Read the model definition and answer for the solid it produces. Units are mm, in the model's axes. A direction names the side the tool comes from. Coordinates: 2 decimals unless noted, no trailing zeros. Loops run counter-clockwise (first coordinate to the right, second up) from the corner with the lowest first, then second, coordinate; pieces in that order, holes last. Notation, with made-up numbers: (61, 54) -> (92, 54) arc R13 ccw to (92, 70) -> close; hole circle Ø4 at (52.25, 33.25). An arc over 180 degrees is marked (long way). Answer in a Markdown table with one row per item.
```python
from build123d import *

# Parameters (mm, degrees)
F1_DEPTH     = 20
F3_D         = 5
F5_T3_DEPTH  = 150
F5_T6_DEPTH  = 40
F5_T9_DEPTH  = 30
F5_T12_DEPTH = 25
F5_T15_DEPTH = 100
F5_T18_DEPTH = 25
F5_T21_DEPTH = 30
F5_T24_DEPTH = 40
F5_T33_DEPTH = 150
F5_T36_DEPTH = 40
F5_T39_DEPTH = 30
F5_T42_DEPTH = 25
F5_T45_DEPTH = 100
F5_T48_DEPTH = 25
F5_T51_DEPTH = 30
F5_T54_DEPTH = 40
F5_T64_DEPTH = 105
F5_T68_DEPTH = 30
F5_T74_DEPTH = 30
F5_T78_DEPTH = 105
F5_T84_DEPTH = 30
F5_T88_DEPTH = 105
F5_T94_DEPTH = 105
F5_T98_DEPTH = 30


# Not quite as in the source:
# - a fillet or chamfer that OpenCascade refuses, or shapes differently, is made with other operations: its cross-section is extruded or revolved along the edge and cut away or added


with BuildPart() as f1:
    # F0 (on Top) → F1 (new body)
    with BuildSketch(Plane.XY):
        Polygon((45.4953936456, 30), (-24.5046063544, 30), (-24.5046063544, 20), (25.4953936456, 20), (25.4953936456, 0), (45.4953936456, 0), align=None)
    extrude(amount=F1_DEPTH)

    # F3 (through all)
    with Locations(Plane.XY.offset(20)):
        with Locations((40.4953936456, 5)):
            Hole(F3_D / 2)

    # F4: F1 across face


with BuildPart() as f1_1:
    add(f1.part)
    add(f1.part.mirror(Plane(origin=(-24.5046063544, 25, 10), x_dir=(0, -1, 0), z_dir=(-1, 0, 0))))

    # F5: fillet of radius 2 on 20 edges, made by hand


with BuildPart() as f5_tool1:
    # F5_s2 → F5_t3 (new body)
    with BuildSketch(Plane.YZ.offset(-99.5046063544)):
        with BuildLine():
            ThreePointArc((30, 18), (29.4142135624, 19.4142135624), (28, 20))
            Line((28, 20), (30, 20))
            Line((30, 20), (30, 18))
        make_face()
    extrude(amount=F5_T3_DEPTH)


with BuildPart() as f5_tool4:
    # F5_s5 → F5_t6 (new body)
    with BuildSketch(Plane.XZ.offset(5)):
        with BuildLine():
            ThreePointArc((-94.5046063544, 18), (-93.9188199167, 19.4142135624), (-92.5046063544, 20))
            Line((-92.5046063544, 20), (-94.5046063544, 20))
            Line((-94.5046063544, 20), (-94.5046063544, 18))
        make_face()
    extrude(amount=-F5_T6_DEPTH)


with BuildPart() as f5_tool7:
    # F5_s8 → F5_t9 (new body)
    with BuildSketch(Plane.YZ.offset(-69.5046063544)):
        with BuildLine():
            ThreePointArc((0, 18), (0.5857864376, 19.4142135624), (2, 20))
            Line((2, 20), (0, 20))
            Line((0, 20), (0, 18))
        make_face()
    extrude(amount=-F5_T9_DEPTH)


with BuildPart() as f5_tool10:
    # F5_s11 → F5_t12 (new body)
    with BuildSketch(Plane.XZ.offset(-20)):
        with BuildLine():
            ThreePointArc((-74.5046063544, 18), (-75.090392792, 19.4142135624), (-76.5046063544, 20))
            Line((-76.5046063544, 20), (-74.5046063544, 20))
            Line((-74.5046063544, 20), (-74.5046063544, 18))
        make_face()
    extrude(amount=F5_T12_DEPTH)


with BuildPart() as f5_tool13:
    # F5_s14 → F5_t15 (new body)
    with BuildSketch(Plane.YZ.offset(-74.5046063544)):
        with BuildLine():
            ThreePointArc((20, 18), (20.5857864376, 19.4142135624), (22, 20))
            Line((22, 20), (20, 20))
            Line((20, 20), (20, 18))
        make_face()
    extrude(amount=F5_T15_DEPTH)


with BuildPart() as f5_tool16:
    # F5_s17 → F5_t18 (new body)
    with BuildSketch(Plane.XZ.offset(-20)):
        with BuildLine():
            ThreePointArc((25.4953936456, 18), (26.0811800833, 19.4142135624), (27.4953936456, 20))
            Line((27.4953936456, 20), (25.4953936456, 20))
            Line((25.4953936456, 20), (25.4953936456, 18))
        make_face()
    extrude(amount=F5_T18_DEPTH)


with BuildPart() as f5_tool19:
    # F5_s20 → F5_t21 (new body)
    with BuildSketch(Plane.YZ.offset(20.4953936456)):
        with BuildLine():
            ThreePointArc((0, 18), (0.5857864376, 19.4142135624), (2, 20))
            Line((2, 20), (0, 20))
            Line((0, 20), (0, 18))
        make_face()
    extrude(amount=F5_T21_DEPTH)


with BuildPart() as f5_tool22:
    # F5_s23 → F5_t24 (new body)
    with BuildSketch(Plane.XZ.offset(5)):
        with BuildLine():
            ThreePointArc((43.4953936456, 20), (44.909607208, 19.4142135624), (45.4953936456, 18))
            Line((45.4953936456, 18), (45.4953936456, 20))
            Line((45.4953936456, 20), (43.4953936456, 20))
        make_face()
    extrude(amount=-F5_T24_DEPTH)


with BuildPart() as f5_tool25:
    # F5_s26 → F5_t27 (revolve)
    with BuildSketch(Plane.XZ.offset(-5)):
        with BuildLine():
            ThreePointArc((42.9953936456, 18), (43.5811800833, 19.4142135624), (44.9953936456, 20))
            Line((44.9953936456, 20), (42.9953936456, 20))
            Line((42.9953936456, 20), (42.9953936456, 18))
        make_face()
    revolve(axis=Axis((40.4953936456, 5, 20), (0, 0, 1)))


with BuildPart() as f5_tool28:
    # F5_s29 → F5_t30 (revolve)
    with BuildSketch(Plane.XZ.offset(-5)):
        with BuildLine():
            ThreePointArc((-92.0046063544, 18), (-92.590392792, 19.4142135624), (-94.0046063544, 20))
            Line((-94.0046063544, 20), (-92.0046063544, 20))
            Line((-92.0046063544, 20), (-92.0046063544, 18))
        make_face()
    revolve(axis=Axis((-89.5046063544, 5, 20), (0, 0, -1)))


with BuildPart() as f5_tool31:
    # F5_s32 → F5_t33 (new body)
    with BuildSketch(Plane.YZ.offset(50.4953936456)):
        with BuildLine():
            ThreePointArc((30, 2), (29.4142135624, 0.5857864376), (28, 0))
            Line((28, 0), (30, 0))
            Line((30, 0), (30, 2))
        make_face()
    extrude(amount=-F5_T33_DEPTH)


with BuildPart() as f5_tool34:
    # F5_s35 → F5_t36 (new body)
    with BuildSketch(Plane.XZ.offset(5)):
        with BuildLine():
            ThreePointArc((-92.5046063544, 0), (-93.9188199167, 0.5857864376), (-94.5046063544, 2))
            Line((-94.5046063544, 2), (-94.5046063544, 0))
            Line((-94.5046063544, 0), (-92.5046063544, 0))
        make_face()
    extrude(amount=-F5_T36_DEPTH)


with BuildPart() as f5_tool37:
    # F5_s38 → F5_t39 (new body)
    with BuildSketch(Plane.YZ.offset(-69.5046063544)):
        with BuildLine():
            ThreePointArc((2, 0), (0.5857864376, 0.5857864376), (0, 2))
            Line((0, 2), (0, 0))
            Line((0, 0), (2, 0))
        make_face()
    extrude(amount=-F5_T39_DEPTH)


with BuildPart() as f5_tool40:
    # F5_s41 → F5_t42 (new body)
    with BuildSketch(Plane.XZ.offset(-20)):
        with BuildLine():
            ThreePointArc((-76.5046063544, 0), (-75.090392792, 0.5857864376), (-74.5046063544, 2))
            Line((-74.5046063544, 2), (-74.5046063544, 0))
            Line((-74.5046063544, 0), (-76.5046063544, 0))
        make_face()
    extrude(amount=F5_T42_DEPTH)


with BuildPart() as f5_tool43:
    # F5_s44 → F5_t45 (new body)
    with BuildSketch(Plane.YZ.offset(25.4953936456)):
        with BuildLine():
            ThreePointArc((22, 0), (20.5857864376, 0.5857864376), (20, 2))
            Line((20, 2), (20, 0))
            Line((20, 0), (22, 0))
        make_face()
    extrude(amount=-F5_T45_DEPTH)


with BuildPart() as f5_tool46:
    # F5_s47 → F5_t48 (new body)
    with BuildSketch(Plane.XZ.offset(-20)):
        with BuildLine():
            ThreePointArc((27.4953936456, 0), (26.0811800833, 0.5857864376), (25.4953936456, 2))
            Line((25.4953936456, 2), (25.4953936456, 0))
            Line((25.4953936456, 0), (27.4953936456, 0))
        make_face()
    extrude(amount=F5_T48_DEPTH)


with BuildPart() as f5_tool49:
    # F5_s50 → F5_t51 (new body)
    with BuildSketch(Plane.YZ.offset(20.4953936456)):
        with BuildLine():
            ThreePointArc((2, 0), (0.5857864376, 0.5857864376), (0, 2))
            Line((0, 2), (0, 0))
            Line((0, 0), (2, 0))
        make_face()
    extrude(amount=F5_T51_DEPTH)


with BuildPart() as f5_tool52:
    # F5_s53 → F5_t54 (new body)
    with BuildSketch(Plane.XZ.offset(5)):
        with BuildLine():
            ThreePointArc((43.4953936456, 0), (44.909607208, 0.5857864376), (45.4953936456, 2))
            Line((45.4953936456, 2), (45.4953936456, 0))
            Line((45.4953936456, 0), (43.4953936456, 0))
        make_face()
    extrude(amount=-F5_T54_DEPTH)


with BuildPart() as f5_tool55:
    # F5_s56 → F5_t57 (revolve)
    with BuildSketch(Plane.XZ.offset(-5)):
        with BuildLine():
            ThreePointArc((44.9953936456, 0), (43.5811800833, 0.5857864376), (42.9953936456, 2))
            Line((42.9953936456, 2), (42.9953936456, 0))
            Line((42.9953936456, 0), (44.9953936456, 0))
        make_face()
    revolve(axis=Axis((40.4953936456, 5, 0), (0, 0, 1)))


with BuildPart() as f5_tool58:
    # F5_s59 → F5_t60 (revolve)
    with BuildSketch(Plane.XZ.offset(-5)):
        with BuildLine():
            ThreePointArc((-94.0046063544, 0), (-92.590392792, 0.5857864376), (-92.0046063544, 2))
            Line((-92.0046063544, 2), (-92.0046063544, 0))
            Line((-92.0046063544, 0), (-94.0046063544, 0))
        make_face()
    revolve(axis=Axis((-89.5046063544, 5, 0), (0, 0, -1)))


with BuildPart() as f5_tool62:
    # F5_s63 → F5_t64 (new body)
    with BuildSketch(Plane.YZ.offset(-79.5046063544)):
        with BuildLine():
            ThreePointArc((20, 18), (20.5857864376, 19.4142135624), (22, 20))
            Line((22, 20), (20, 20))
            Line((20, 20), (20, 18))
        make_face()
    extrude(amount=F5_T64_DEPTH)

    split(bisect_by=Plane.YZ.offset(-74.5046063544), keep=Keep.BOTTOM)


with BuildPart() as f5_tool66:
    # F5_s67 → F5_t68 (new body)
    with BuildSketch(Plane.XZ.offset(-25)):
        with BuildLine():
            ThreePointArc((-74.5046063544, 18), (-75.090392792, 19.4142135624), (-76.5046063544, 20))
            Line((-76.5046063544, 20), (-74.5046063544, 20))
            Line((-74.5046063544, 20), (-74.5046063544, 18))
        make_face()
    extrude(amount=F5_T68_DEPTH)

    split(bisect_by=Plane.XZ.offset(-20), keep=Keep.BOTTOM)


with BuildPart() as f5_tool62_1:
    add(f5_tool62.part)

    # F5_t70: intersect F5_tool66
    add(f5_tool66.part, mode=Mode.INTERSECT)


with BuildPart() as f5_tool72:
    # F5_s73 → F5_t74 (new body)
    with BuildSketch(Plane.XZ.offset(-25)):
        with BuildLine():
            ThreePointArc((25.4953936456, 18), (26.0811800833, 19.4142135624), (27.4953936456, 20))
            Line((27.4953936456, 20), (25.4953936456, 20))
            Line((25.4953936456, 20), (25.4953936456, 18))
        make_face()
    extrude(amount=F5_T74_DEPTH)

    split(bisect_by=Plane.XZ.offset(-20), keep=Keep.BOTTOM)


with BuildPart() as f5_tool76:
    # F5_s77 → F5_t78 (new body)
    with BuildSketch(Plane.YZ.offset(-74.5046063544)):
        with BuildLine():
            ThreePointArc((20, 18), (20.5857864376, 19.4142135624), (22, 20))
            Line((22, 20), (20, 20))
            Line((20, 20), (20, 18))
        make_face()
    extrude(amount=F5_T78_DEPTH)

    split(bisect_by=Plane.YZ.offset(25.4953936456), keep=Keep.TOP)


with BuildPart() as f5_tool72_1:
    add(f5_tool72.part)

    # F5_t80: intersect F5_tool76
    add(f5_tool76.part, mode=Mode.INTERSECT)


with BuildPart() as f5_tool82:
    # F5_s83 → F5_t84 (new body)
    with BuildSketch(Plane.XZ.offset(-25)):
        with BuildLine():
            ThreePointArc((-76.5046063544, 0), (-75.090392792, 0.5857864376), (-74.5046063544, 2))
            Line((-74.5046063544, 2), (-74.5046063544, 0))
            Line((-74.5046063544, 0), (-76.5046063544, 0))
        make_face()
    extrude(amount=F5_T84_DEPTH)

    split(bisect_by=Plane.XZ.offset(-20), keep=Keep.BOTTOM)


with BuildPart() as f5_tool86:
    # F5_s87 → F5_t88 (new body)
    with BuildSketch(Plane.YZ.offset(25.4953936456)):
        with BuildLine():
            ThreePointArc((22, 0), (20.5857864376, 0.5857864376), (20, 2))
            Line((20, 2), (20, 0))
            Line((20, 0), (22, 0))
        make_face()
    extrude(amount=-F5_T88_DEPTH)

    split(bisect_by=Plane.YZ.offset(-74.5046063544), keep=Keep.BOTTOM)


with BuildPart() as f5_tool82_1:
    add(f5_tool82.part)

    # F5_t90: intersect F5_tool86
    add(f5_tool86.part, mode=Mode.INTERSECT)


with BuildPart() as f5_tool92:
    # F5_s93 → F5_t94 (new body)
    with BuildSketch(Plane.YZ.offset(30.4953936456)):
        with BuildLine():
            ThreePointArc((22, 0), (20.5857864376, 0.5857864376), (20, 2))
            Line((20, 2), (20, 0))
            Line((20, 0), (22, 0))
        make_face()
    extrude(amount=-F5_T94_DEPTH)

    split(bisect_by=Plane.YZ.offset(25.4953936456), keep=Keep.TOP)


with BuildPart() as f5_tool96:
    # F5_s97 → F5_t98 (new body)
    with BuildSketch(Plane.XZ.offset(-25)):
        with BuildLine():
            ThreePointArc((27.4953936456, 0), (26.0811800833, 0.5857864376), (25.4953936456, 2))
            Line((25.4953936456, 2), (25.4953936456, 0))
            Line((25.4953936456, 0), (27.4953936456, 0))
        make_face()
    extrude(amount=F5_T98_DEPTH)

    split(bisect_by=Plane.XZ.offset(-20), keep=Keep.BOTTOM)


with BuildPart() as f5_tool92_1:
    add(f5_tool92.part)

    # F5_t100: intersect F5_tool96
    add(f5_tool96.part, mode=Mode.INTERSECT)


with BuildPart() as f1_2:
    add(f1_1.part)

    # F5_t101: cut F5_tool1, F5_tool4, F5_tool7, F5_tool10, F5_tool13, F5_tool16, F5_tool19, F5_tool22, F5_tool25, F5_tool28, F5_tool31, F5_tool34, F5_tool37, F5_tool40, F5_tool43, F5_tool46, F5_tool49, F5_tool52, F5_tool55, F5_tool58, F5_tool62, F5_tool72, F5_tool82, F5_tool92
    add([f5_tool1.part, f5_tool4.part, f5_tool7.part, f5_tool10.part, f5_tool13.part, f5_tool16.part, f5_tool19.part, f5_tool22.part, f5_tool25.part, f5_tool28.part, f5_tool31.part, f5_tool34.part, f5_tool37.part, f5_tool40.part, f5_tool43.part, f5_tool46.part, f5_tool49.part, f5_tool52.part, f5_tool55.part, f5_tool58.part, f5_tool62_1.part, f5_tool72_1.part, f5_tool82_1.part, f5_tool92_1.part], mode=Mode.SUBTRACT)


solid = f1_2.part
```
1. A tool of negligible diameter and unlimited length cuts with its end or side. For faces 1 (the flat face through (-24, 20, 10)), 2 (the flat face through (-24, 24, 20)), from which of +Z, -Z, +X, -X, +Y, -Y can it reach the whole face along a straight path? Write none if from no direction.
A:
| item | result |
|---|---|
| face 1 | +Z, -Z, -Y |
| face 2 | +Z, +X, -X, +Y, -Y |
2. Find the intervals of material crossed by probe 1 along X at (y, z) = (15, 10); probe 2 along Y at (x, z) = (-42, 2.25); probe 3 along X at (y, z) = (9, 19), in increasing order.
A:
| item | result |
|---|---|
| probe 1 | x = -94.5 to -74.5, 25.5 to 45.5 |
| probe 2 | y = 20 to 30 |
| probe 3 | x = -94.24 to -74.77, 25.76 to 45.23 |
3. Given pin 1 Ø4.5 at (x, y) = (40.5, 5) entering from -Z; pin 2 Ø10 at (x, z) = (-35, 5) entering from -Y; pin 3 Ø6.5 at (x, y) = (-89.5, 5) entering from -Z, each flat-ended and moving along its own axis, determine where each tip first touches the part or whether it passes through.
A:
| item | result |
|---|---|
| pin 1 | passes through |
| pin 2 | stops at y = 20 |
| pin 3 | stops at z = 0.44 |
4. A cutting plane is placed at C-C on x = 16. Give the vertices of the cut face in (y, z), and give its area (3 significant figures).
A:
| item | result |
|---|---|
| outline | (20, 2) arc R2 ccw to (22, 0) -> (28, 0) arc R2 ccw to (30, 2) -> (30, 18) arc R2 ccw to (28, 20) -> (22, 20) arc R2 ccw to (20, 18) -> close |
| area | 197 mm2 |
5. The mould has two halves that part along X. Classify faces 3 (the flat face through (-24, 24, 0)), 4 (the flat face through (-94.505, 15, 10)), 5 (the cylindrical face through (38.11, 5.75, 9.89)): pulls with the +X half, pulls with the -X half, needs draft (parallel to the pull), parting line crosses it, or undercut.
A:
| item | result |
|---|---|
| face 3 | needs draft |
| face 4 | pulls with the -X half |
| face 5 | undercut |
6. A cutting plane is placed at D-D on y = 5. Give the vertices of the cut face in (x, z), and give its area (3 significant figures).
A:
| item | result |
|---|---|
| outline | (-94.5, 2) arc R2 ccw to (-93.25, 0.15) arc R2 ccw to (-92, 2) -> (-92, 18) arc R2 ccw to (-93.25, 19.85) arc R2 ccw to (-94.5, 18) -> close; (-87, 2) arc R2 ccw to (-85, 0) -> (-76.5, 0) arc R2 ccw to (-74.5, 2) -> (-74.5, 18) arc R2 ccw to (-76.5, 20) -> (-85, 20) arc R2 ccw to (-87, 18) -> close; (25.5, 2) arc R2 ccw to (27.5, 0) -> (36, 0) arc R2 ccw to (38, 2) -> (38, 18) arc R2 ccw to (36, 20) -> (27.5, 20) arc R2 ccw to (25.5, 18) -> close; (43, 2) arc R2 ccw to (44.25, 0.15) arc R2 ccw to (45.5, 2) -> (45.5, 18) arc R2 ccw to (44.25, 19.85) arc R2 ccw to (43, 18) -> close |
| area | 587 mm2 |
7. A cutting plane is placed at B-B on z = 3.5. Give the vertices of the cut face in (x, y), and give its area (3 significant figures).
A:
| item | result |
|---|---|
| outline | (-94.5, 0) -> (-74.5, 0) -> (-74.5, 20) -> (25.5, 20) -> (25.5, 0) -> (45.5, 0) -> (45.5, 30) -> (-94.5, 30) -> close; hole circle Ø5 at (-89.5, 5); hole circle Ø5 at (40.5, 5) |
| area | 2,160 mm2 |
8. A cutting plane is placed at A-A on y = 13.5. Give the vertices of the cut face in (x, z).
A:
| item | result |
|---|---|
| outline | (-94.5, 2) arc R2 ccw to (-92.5, 0) -> (-76.5, 0) arc R2 ccw to (-74.5, 2) -> (-74.5, 18) arc R2 ccw to (-76.5, 20) -> (-92.5, 20) arc R2 ccw to (-94.5, 18) -> close; (25.5, 2) arc R2 ccw to (27.5, 0) -> (43.5, 0) arc R2 ccw to (45.5, 2) -> (45.5, 18) arc R2 ccw to (43.5, 20) -> (27.5, 20) arc R2 ccw to (25.5, 18) -> close |
